Autodesk Inventor part; units mm, degrees
ref_plane "YZ Plane" through (0, 0, 0) normal (1, 0, 0) x (0, 1, 0)
ref_plane "XZ Plane" through (0, 0, 0) normal (0, 1, 0) x (-1, 0, 0)
ref_plane "XY Plane" through (0, 0, 0) normal (0, 0, 1) x (1, 0, 0)
sketch "スケッチ1" plane through (0, 0, 0) normal (0, 0, 1) x (1, 0, 0)
  line L0 (-15, 5.75) -> (-15, -5.75)
  line L1 (-15, -5.75) -> (-12, -5.75)
  line L2 (-12, -5.75) -> (-12, -3.65)
  line L3 (-12, -3.65) -> (-7, -3.65)
  line L4 (-7, -3.65) -> (-7, -3.75)
  line L5 (-7, -3.75) -> (-5, -3.75)
  line L6 (-5, -3.75) -> (-5, 3.75)
  line L7 (0, 0) -> (-15, 0) construction
  line L8 (-15, 5.75) -> (-12, 5.75)
  line L9 (-12, 5.75) -> (-12, 3.65)
  line L10 (-12, 3.65) -> (-7, 3.65)
  line L11 (-7, 3.65) -> (-7, 3.75)
  line L12 (-7, 3.75) -> (-5, 3.75)
  line L13 (0, 0) -> (0, 5.75) construction
  point P0 (-5, 0)
  dimension "d0" = 11.5
  dimension "d1" = 15
  dimension "d2" = 5
  dimension "d3" = 0.1
  dimension "d4" = 2
  dimension "d5" = 3
  dimension "d6" = 2
revolve "回転1" add sketch "スケッチ1" angle 360 about axis through (0, 0, 0) along (0, 1, 0)
properties part number "Gbear_30_10" material "ステンレス鋼"
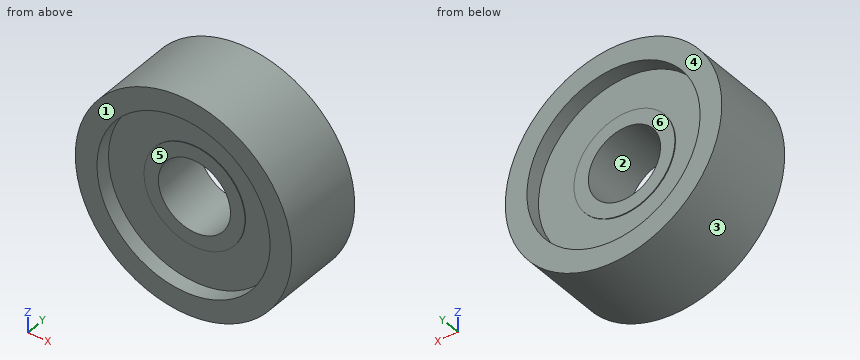
Could you check a few things on this model? Use its own coordinates, in mm. Face numbers are marked on the shaded views. A direction names the side the tool comes from. Coordinates: 2 decimals unless noted, no trailing zeros. Loops run counter-clockwise (first coordinate to the right, second up) from the corner with the lowest first, then second, coordinate; pieces in that order, holes last.
1. I need wall thicknesses on L1, parallel to Z at x = 0, y = 4.6; L2, parallel to Z at x = 0, y = -1.25; L3, parallel to X at y = 4, z = 1.75. Which ranges of each line are inside material? Lowest first, please.
2. Imagine slicing it at B-B (z = 0). Please give me the cut outline in (x, y), and give its area (3 significant figures).
3. For P1, Ø1, axis at y = -2, z = -3, coming from the -X side; P2, Ø7, axis at x = 1.5, z = -2, coming from the +Y side; P3, Ø1.5, axis at x = 4.5, y = -2.5, coming from the -Z side, each with a flat end and sliding along its axis, tell me the tip position at first contact or that it passes through.
4. Imagine slicing it at A-A (x = 0). Please give me the cut outline in (y, z), and give its area (3 significant figures).
5. Imagine slicing it at D-D (x = 10.25). Please give me the cut outline in (y, z), and give its area (3 significant figures).
6. Imagine slicing it at C-C (y = 0). Please give me the cut outline in (x, z).
7. For the marked faces 4, 5 and 6, which set-ups out of +Z, -Z, +X, -X, +Y, -Y let a thin tool reach every point of the face, with its end or its side?
8. We'd pull the mould along Z, two halves only. Please class the marked faces 1, 2 and 3: released by +Z, released by -Z, zero draft, split by the parting line, or undercut.
Computed values:
1. L1: z = -15 to -12, 12 to 15
1. L2: z = -15 to -5, 5 to 15
1. L3: x = -14.9 to -11.87, 11.87 to 14.9
2. outline: (-15, -5.75) - (-12, -5.75) - (-12, -3.65) - (-7, -3.65) - (-7, -3.75) - (-5, -3.75) - (-5, 3.75) - (-7, 3.75) - (-7, 3.65) - (-12, 3.65) - (-12, 5.75) - (-15, 5.75) - close; (5, -3.75) - (7, -3.75) - (7, -3.65) - (12, -3.65) - (12, -5.75) - (15, -5.75) - (15, 5.75) - (12, 5.75) - (12, 3.65) - (7, 3.65) - (7, 3.75) - (5, 3.75) - close
2. area: 172 mm2
3. P1: stops at x = -14.79
3. P2: stops at y = 3.75
3. P3: stops at z = -14.52
4. outline: (-5.75, -15) - (5.75, -15) - (5.75, -12) - (3.65, -12) - (3.65, -7) - (3.75, -7) - (3.75, -5) - (-3.75, -5) - (-3.75, -7) - (-3.65, -7) - (-3.65, -12) - (-5.75, -12) - close; (-5.75, 12) - (-3.65, 12) - (-3.65, 7) - (-3.75, 7) - (-3.75, 5) - (3.75, 5) - (3.75, 7) - (3.65, 7) - (3.65, 12) - (5.75, 12) - (5.75, 15) - (-5.75, 15) - close
4. area: 172 mm2
5. outline: (-5.75, -10.95) - (5.75, -10.95) - (5.75, -6.24) - (3.65, -6.24) - (3.65, 6.24) - (5.75, 6.24) - (5.75, 10.95) - (-5.75, 10.95) - (-5.75, 6.24) - (-3.65, 6.24) - (-3.65, -6.24) - (-5.75, -6.24) - close
5. area: 199 mm2
6. outline: circle Ø30 at (0, 0); hole circle Ø10 at (0, 0)
7. face 4: +Z, -Z, +X, -X, +Y
7. face 5: -Y
7. face 6: +Y
8. face 1: zero draft
8. face 2: undercut
8. face 3: split by the parting line
